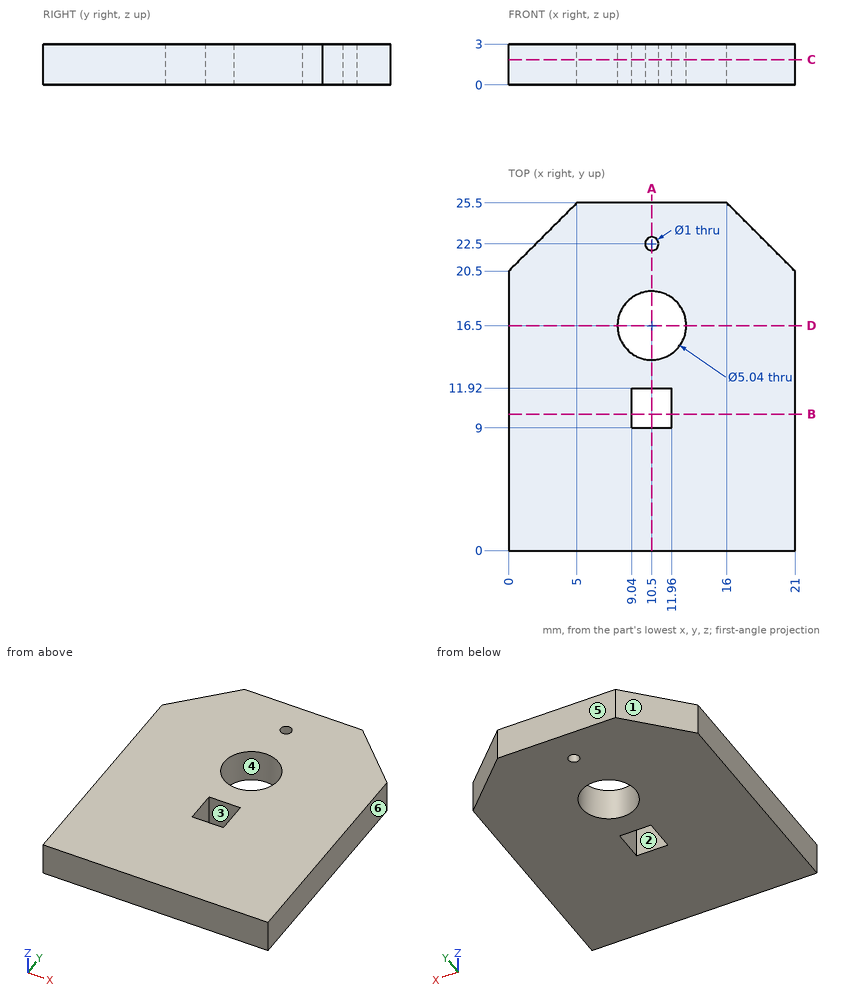
Verification items for this drawing (mm, ordinates from the low corner). A direction names the side the tool comes from. Give positions to 0.01 mm unless a question says otherwise; leave off trailing zeros. Write each loop counter-clockwise with the first axis right and the second up, starting at its lowest first coordinate (ties: lowest second). Pieces come first, ordered by that corner, then holes. Notation, with made-up numbers: (41.5, 69.5) - (51.5, 69.5) arc R13 cw to (51.5, 81.5) - close; hole circle Ø5 at (12.25, 58). An arc over 180 degrees is marked (long way). Answer as a JSON object with one key per item and string values. Group by question number.
1) Sectioned sample at C-C (z = 1.85). Record the cut outline in (x, y), then the cut area to 3 significant figures.
2) Depth check by flat-ended pin: P1, Ø8, axis at x = 10.5, y = 16.5, coming from the +Z side. Enter the tip coordinate at first touch or a pass-through.
3) Access from +Z, -Z, +X, -X, +Y, -Y to the whole of each face (thin tool, end or side, straight path). Record for the marked faces 1 and 2.
4) Sectioned sample at B-B (y = 10). Record the cut outline in (x, z).
5) Sectioned sample at A-A (x = 10.5). Record the cut outline in (y, z).
6) Sectioned sample at D-D (y = 16.5). Record the cut outline in (x, z).
7) Thickness scan on probe 1 along Y at (x, z) = (10.5, 0.95); probe 2 along X at (y, z) = (9.75, 2.5); probe 3 along Y at (x, z) = (11.25, 0.1). Record the ranges inside material, lowest first. Write a range as from..to.
8) Release check for a two-part mould opening along Y. For the marked faces 3, 4, 5 and 6 record: pulls with the +Y half, pulls with the -Y half, needs draft (parallel to the pull), parting line crosses it, or undercut.
Geometry results:
{
 "1": {"outline": "(0, 0) - (21, 0) - (21, 20.5) - (16, 25.5) - (5, 25.5) - (0, 20.5) - close; hole circle Ø5.04 at (10.5, 16.5); hole (9.04, 9) - (11.96, 9) - (11.96, 11.92) - (9.04, 11.92) - close; hole circle Ø1 at (10.5, 22.5)", "area": "481 mm^2"},
 "2": {"P1": "stops at z = 3"},
 "3": {"face 1": "+Z, -Z, -X, +Y", "face 2": "+Z, -Z"},
 "4": {"outline": "(0, 0) - (9.04, 0) - (9.04, 3) - (0, 3) - close; (11.96, 0) - (21, 0) - (21, 3) - (11.96, 3) - close"},
 "5": {"outline": "(0, 0) - (9, 0) - (9, 3) - (0, 3) - close; (11.92, 0) - (13.98, 0) - (13.98, 3) - (11.92, 3) - close; (19.02, 0) - (22, 0) - (22, 3) - (19.02, 3) - close; (23, 0) - (25.5, 0) - (25.5, 3) - (23, 3) - close"},
 "6": {"outline": "(0, 0) - (7.98, 0) - (7.98, 3) - (0, 3) - close; (13.02, 0) - (21, 0) - (21, 3) - (13.02, 3) - close"},
 "7": {"probe 1": "y = 0..9, 11.92..13.98, 19.02..22, 23..25.5", "probe 2": "x = 0..9.04, 11.96..21", "probe 3": "y = 0..9, 11.92..14.09, 18.91..25.5"},
 "8": {"face 3": "undercut", "face 4": "undercut", "face 5": "pulls with the +Y half", "face 6": "needs draft"}
}
